from build123d import *

# Parameters (mm, degrees)
SKETCH1_W           = 200
SKETCH1_H           = 100
BOSS_EXTRUDE1_DEPTH = 20
SKETCH2_R           = 14
CUT_EXTRUDE1_DEPTH  = 15
SKETCH4_R           = 5
CUT_EXTRUDE3_DEPTH  = 114.578166916


with BuildPart() as part:
    # Sketch1 → Boss-Extrude1 (new body)
    with BuildSketch(Plane.XY):
        Rectangle(SKETCH1_W, SKETCH1_H)
    extrude(amount=BOSS_EXTRUDE1_DEPTH)

    # Sketch2 → Cut-Extrude1 (cut)
    with BuildSketch(Plane.XY.offset(20)):
        with Locations((-50, 0)):
            Circle(SKETCH2_R)
        with Locations(Location((50, 0, 0), (0, 0, 180))):
            Circle(SKETCH2_R)
    extrude(amount=-CUT_EXTRUDE1_DEPTH, mode=Mode.SUBTRACT)

    # Sketch4 → Cut-Extrude3 (cut, through all)
    with BuildSketch(Plane(origin=(0, 0, 0), x_dir=(-1, 0, 0), z_dir=(0, 0, -1))):
        with Locations((-80, -29.75)):
            Circle(SKETCH4_R)
        with Locations((80, -29.75)):
            Circle(SKETCH4_R)
    extrude(amount=-CUT_EXTRUDE3_DEPTH, mode=Mode.SUBTRACT)


solid = part.part
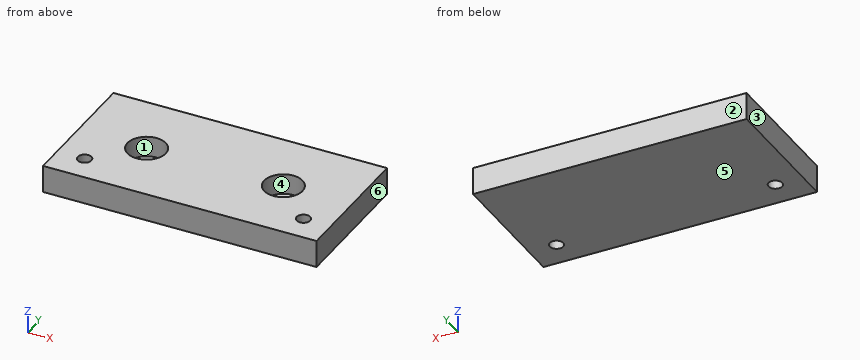
Part model, mm, in its own coordinate system. Face numbers are marked on the shaded views. A direction names the side the tool comes from. Give positions to 0.01 mm unless a question says otherwise; leave off trailing zeros. Loops run counter-clockwise (first coordinate to the right, second up) from the corner with the lowest first, then second, coordinate; pieces in that order, holes last. Notation, with made-up numbers: M -8,61.25 L 15,61.25 A17 ccw 15,70.25 Z; hole C -32,70 d7. An arc over 180 degrees is marked long. Put each result on its own line as item: value. Start each with the question number.
1) Pull direction X, two halves, no side cores. Call the marked faces 3, 4, 5 and 6: +X half, -X half, draft (parallel to the pull), parting line (faces both ways), or undercut.
2) Probe probe 1 along Y at (x, z) = (50, 5.25); probe 2 along Y at (x, z) = (80, 4); probe 3 along X at (y, z) = (-7, 14.75). List the from-to ranges inside material, lowest first.
3) Saw through at C-C (z = 11). List the corners of the cut face in (x, y).
4) Saw through at A-A (y = -29.75). List the corners of the cut face in (x, z).
5) Saw through at D-D (x = 50). List the corners of the cut face in (y, z), then the cut area to 3 significant figures.
6) Saw through at B-B (x = 80). List the corners of the cut face in (y, z), then the cut area to 3 significant figures.
7) Flat gauge pin, fed straight in: pin 1 (8 mm diameter, centred on x = 80, y = -29.75, fed in from +Z). Where does the tip first touch, or does it go through?
8) 3-axis set-ups, long thin cutter, end or side, ignore diameter. For the marked faces 1 and 2: which of +Z, -Z, +X, -X, +Y, -Y reach the whole face in a straight line?
Numbers:
1. face 3: -X half
1. face 4: undercut
1. face 5: draft
1. face 6: +X half
2. probe 1: -50 to -14, 14 to 50
2. probe 2: -50 to -34.75, -24.75 to 50
2. probe 3: -100 to -62.12, -37.88 to 37.88, 62.12 to 100
3. outline: M -100,-50 L 100,-50 L 100,50 L -100,50 Z; hole C -80,-29.75 d10; hole C -50,0 d28; hole C 50,0 d28; hole C 80,-29.75 d10
4. outline: M -100,0 L -85,0 L -85,20 L -100,20 Z; M -75,0 L 75,0 L 75,20 L -75,20 Z; M 85,0 L 100,0 L 100,20 L 85,20 Z
5. outline: M -50,0 L 50,0 L 50,20 L 14,20 L 14,5 L -14,5 L -14,20 L -50,20 Z
5. area: 1,580 mm^2
6. outline: M -50,0 L -34.75,0 L -34.75,20 L -50,20 Z; M -24.75,0 L 50,0 L 50,20 L -24.75,20 Z
6. area: 1,800 mm^2
7. pin 1: through
8. face 1: +Z
8. face 2: +Z, -Z, +X, -X, +Y
